Geometry check sheet. Reference: the model listing, model coordinates, mm. A direction names the side the tool comes from. Round coordinates to 2 decimals unless told otherwise and drop trailing zeros. Write each loop counter-clockwise with the first axis right and the second up, starting at its lowest first coordinate (ties: lowest second). Pieces come first, ordered by that corner, then holes.
from build123d import *

# Parameters (mm, degrees)
F0_W      = 24
F0_H      = 2
F0_W_2    = 22.5
F1_DEPTH  = 3
F2_R      = 10
F3_R      = 1.5
F4_DEPTH  = 2
F5_DEPTH  = 6
F6_R      = 1.9
F6_R_2    = 1.5
F7_DEPTH  = 1
F9_W      = 1
F9_H      = 3.4420455096
F9_W_2    = 3.6737932861
F9_H_2    = 0.5
F9_W_3    = 2.2944888771
F9_H_3    = 2.8
F9_W_4    = 3.9643547535
F10_DEPTH = 6


# Not quite as in the source:
# - a fillet or chamfer that OpenCascade refuses, or shapes differently, is made with other operations: its cross-section is extruded or revolved along the edge and cut away or added


with BuildPart() as f1:
    # F0 (on Top) → F1 (new body)
    with BuildSketch(Plane.XY):
        with Locations((-41.5, 1)):
            Rectangle(F0_W, F0_H)
        Polygon((-29.5, 2), (-29.5, 0), (-22.5, 6), (-22.5, 8), align=None)
        with Locations((-11.25, 7)):
            Rectangle(F0_W_2, F0_H)
        with Locations((11.25, 7)):
            Rectangle(F0_W_2, F0_H)
        Polygon((22.5, 8), (22.5, 6), (29.5, 0), (29.5, 2), align=None)
        with Locations((41.5, 1)):
            Rectangle(F0_W, F0_H)
    extrude(amount=F1_DEPTH)

    # F2
    f2_edges = [f1.edges().sort_by_distance(p)[0] for p in [
        (-29.5, 2, 1.5),
        (-22.5, 8, 1.5),
        (22.5, 8, 1.5),
        (29.5, 2, 1.5),
        (29.5, 0, 1.5),
        (22.5, 6, 1.5),
        (-22.5, 6, 1.5),
        (-29.5, 0, 1.5),
    ]]
    fillet(f2_edges, radius=F2_R)

    # F3 (on face) → F4 (join, through all)
    with BuildSketch(Plane.XZ):
        with BuildLine():
            Line((-53.5, 0), (-53.5, 3))
            ThreePointArc((-53.5, 3), (-55, 1.5), (-53.5, 0))
        make_face()
        with Locations((53.5, 1.5)):
            Circle(F3_R)
    extrude(amount=-F4_DEPTH)

    # F3 (on face) → F5 (join)
    with BuildSketch(Plane.XZ):
        with BuildLine():
            Line((-53.5, 0), (-53.5, 3))
            ThreePointArc((-53.5, 3), (-55, 1.5), (-53.5, 0))
        make_face()
        with BuildLine():
            ThreePointArc((-53.5, 0), (-52.4393398282, 0.4393398282), (-52, 1.5))
            ThreePointArc((-52, 1.5), (-52.4393398282, 2.5606601718), (-53.5, 3))
            Line((-53.5, 3), (-53.5, 0))
        make_face()
        with Locations((53.5, 1.5)):
            Circle(F3_R)
    extrude(amount=F5_DEPTH)

    # F6 (on face) → F7 (join)
    with BuildSketch(Plane.XZ.offset(6)):
        with Locations((-53.5, 1.5)):
            Circle(F6_R)
        with Locations((-53.5, 1.5)):
            Circle(F6_R_2, mode=Mode.SUBTRACT)
        with Locations((53.5, 1.5)):
            Circle(F6_R)
    extrude(amount=-F7_DEPTH)

    # F8: fillet of radius 0.5 on 4 edges, made by hand

    # F8_s1 → F8_t2 (revolve, cut)
    with BuildSketch(Plane.XY.offset(1.5)):
        with BuildLine():
            ThreePointArc((-51.6, -5.5), (-51.7464466094, -5.8535533906), (-52.1, -6))
            Line((-52.1, -6), (-51.6, -6))
            Line((-51.6, -6), (-51.6, -5.5))
        make_face()
    revolve(axis=Axis((-53.5, -6, 1.5), (0, -1, 0)), mode=Mode.SUBTRACT)

    # F8_s3 → F8_t4 (revolve, cut)
    with BuildSketch(Plane.XY.offset(1.5)):
        with BuildLine():
            ThreePointArc((-52, -5), (-51.7127016654, -5.1736701825), (-51.6, -5.4898979486))
            Line((-51.6, -5.4898979486), (-51.6, -5))
            Line((-51.6, -5), (-52, -5))
        make_face()
    revolve(axis=Axis((-53.5, -5, 1.5), (0, -1, 0)), mode=Mode.SUBTRACT)

    # F8_s5 → F8_t6 (revolve, cut)
    with BuildSketch(Plane.XY.offset(1.5)):
        with BuildLine():
            ThreePointArc((55, -5), (55.2872983346, -5.1736701825), (55.4, -5.4898979486))
            Line((55.4, -5.4898979486), (55.4, -5))
            Line((55.4, -5), (55, -5))
        make_face()
    revolve(axis=Axis((53.5, -5, 1.5), (0, -1, 0)), mode=Mode.SUBTRACT)

    # F8_s7 → F8_t8 (revolve, cut)
    with BuildSketch(Plane.XY.offset(1.5)):
        with BuildLine():
            ThreePointArc((55.4, -5.5), (55.2535533906, -5.8535533906), (54.9, -6))
            Line((54.9, -6), (55.4, -6))
            Line((55.4, -6), (55.4, -5.5))
        make_face()
    revolve(axis=Axis((53.5, -6, 1.5), (0, -1, 0)), mode=Mode.SUBTRACT)

    # F9 (on face) → F10 (cut, through all)
    with BuildSketch(Plane.XZ.offset(6)):
        with Locations((-53.5, -2.1210227548)):
            Rectangle(F9_W, F9_H)
        with Locations((-55.836896643, -0.15)):
            Rectangle(F9_W_2, F9_H_2)
        with Locations((-53.5, -0.15)):
            Rectangle(F9_W, F9_H_2)
        with Locations((-51.8527555615, -0.15)):
            Rectangle(F9_W_3, F9_H_2)
        with Locations((-53.5, 1.5)):
            Rectangle(F9_W, F9_H_3)
        with Locations((-55.9821773767, 3.15)):
            Rectangle(F9_W_4, F9_H_2)
        with Locations((-53.5, 3.15)):
            Rectangle(F9_W, F9_H_2)
        with Locations((-51.8527555615, 3.15)):
            Rectangle(F9_W_3, F9_H_2)
        with Locations((-53.5, 5.1210227548)):
            Rectangle(F9_W, F9_H)
        with Locations((55.836896643, -0.15)):
            Rectangle(F9_W_2, F9_H_2)
        with Locations((53.5, -2.1210227548)):
            Rectangle(F9_W, F9_H)
        with Locations((53.5, -0.15)):
            Rectangle(F9_W, F9_H_2)
        with Locations((53.5, 1.5)):
            Rectangle(F9_W, F9_H_3)
        with Locations((51.8527555615, -0.15)):
            Rectangle(F9_W_3, F9_H_2)
        with Locations((55.9821773767, 3.15)):
            Rectangle(F9_W_4, F9_H_2)
        with Locations((53.5, 3.15)):
            Rectangle(F9_W, F9_H_2)
        with Locations((51.8527555615, 3.15)):
            Rectangle(F9_W_3, F9_H_2)
        with Locations((53.5, 5.1210227548)):
            Rectangle(F9_W, F9_H)
    extrude(amount=-F10_DEPTH, mode=Mode.SUBTRACT)


solid = f1.part
1. Depth check by flat-ended pin: pin 1 Ø5 at (x, y) = (-35, 3) entering from +Z; pin 2 Ø0.6 at (x, y) = (54.5, -2.5) entering from +Z; pin 3 Ø0.8 at (y, z) = (-4, 1) entering from -X; pin 4 Ø0.6 at (x, y) = (-52.5, -4) entering from -Z. Enter the tip coordinate at first touch or a pass-through.
2. Section check A-A (y = -2.75). State how many separate pieces and enclosed holes the cut face has, plus the area to 3 significant figures.
3. Release check for a two-part mould opening along Y. For faces 6 (the face through (52, -2.5, 1.5)), 7 (the face through (-44, 2, 2)), 8 (the face through (-55, -1.5, 1.5)), 9 (the face through (-22.32, 5.36, 1.52)) record: +Y half, -Y half, draft (parallel to the pull), parting line (faces both ways), or undercut.
4. Scan lines: line 1 along X through (y, z) = (-1.75, 0.7); line 2 along X through (y, z) = (-4.75, 1.3); line 3 along Y through (x, z) = (37, 1.5). Record each from-to range of solid material in increasing order.
5. Access from +Z, -Z, +X, -X, +Y, -Y to the whole of each face (thin tool, end or side, straight path). Record for faces 1 (the face through (0, 6, 1)), 2 (the face through (44, 2, 1)), 3 (the face through (-29.68, 2.64, 1.52)), 4 (the face through (55, -1.5, 1.5)), 5 (the face through (-0.2, 6.4, 3)).
6. Section check B-B (x = 31). Record the cut outline in (y, z), plus the area to 3 significant figures.
Results below:
1. pin 1: stops at z = 3
1. pin 2: stops at z = 2.83
1. pin 3: stops at x = -55
1. pin 4: stops at z = 0.17
2. separate pieces: 4
2. enclosed holes: 0
2. area: 8.25 mm2
3. face 6: undercut
3. face 7: +Y half
3. face 8: draft
3. face 9: -Y half
4. line 1: x = -54.77 to -54, -53 to -52.23, 52.23 to 53, 54 to 54.77
4. line 2: x = -54.99 to -54, -53 to -52.01, 52.01 to 53, 54 to 54.99
4. line 3: y = 0 to 2
5. face 1: +Z, -Z, -Y
5. face 2: +Z, -Z, +X, +Y
5. face 3: +Z, -Z, -X, +Y
5. face 4: +X, +Y
5. face 5: +Z, +X, -X, +Y, -Y
6. outline: (0.24, 0) - (2.24, 0) - (2.24, 3) - (0.24, 3) - close
6. area: 6.00 mm2
